Check sheet for the drawn part. Datum: minimum x, y, z corner. Units: mm. Coordinates: 2 decimals unless noted, no trailing zeros. Loops run counter-clockwise (first coordinate to the right, second up) from the corner with the lowest first, then second, coordinate; pieces in that order, holes last. Notation, with made-up numbers: (23.5, 4) - (30.5, 4) arc R18 cw to (30.5, 18) - close; hole circle Ø7 at (71, 65). An arc over 180 degrees is marked (long way). Answer as CSV lines item,"result". Start each with the question number.
1. Cross-section at B-B (y = 66). Enter the section's corners in (x, z).
2. Cross-section at C-C (z = 530). Enter the section's corners in (x, y), plus the area to 3 significant figures.
3. Cross-section at D-D (y = 212). Enter the section's corners in (x, z).
4. Gauge pin test, flat ends, axial feed: P1, Ø12.5, axis at x = 72.5, y = 177, coming from the +Z side; P2, Ø12, axis at x = 364.5, y = 23, coming from the -Z side; P3, Ø15, axis at x = 171.5, y = 196, coming from the +Z side. Record the tip position at first contact, or that the pin passes through.
5. Material ranges on line 1 (X direction, y = 44.5, z = 597.5); line 2 (X direction, y = 145.5, z = 645.5); line 3 (Z direction, x = 68.5, y = 183.5), recorded low to high. Write a range as [from, to].
6. Cross-section at A-A (x = 52). Enter the section's corners in (y, z), plus the area to 3 significant figures.
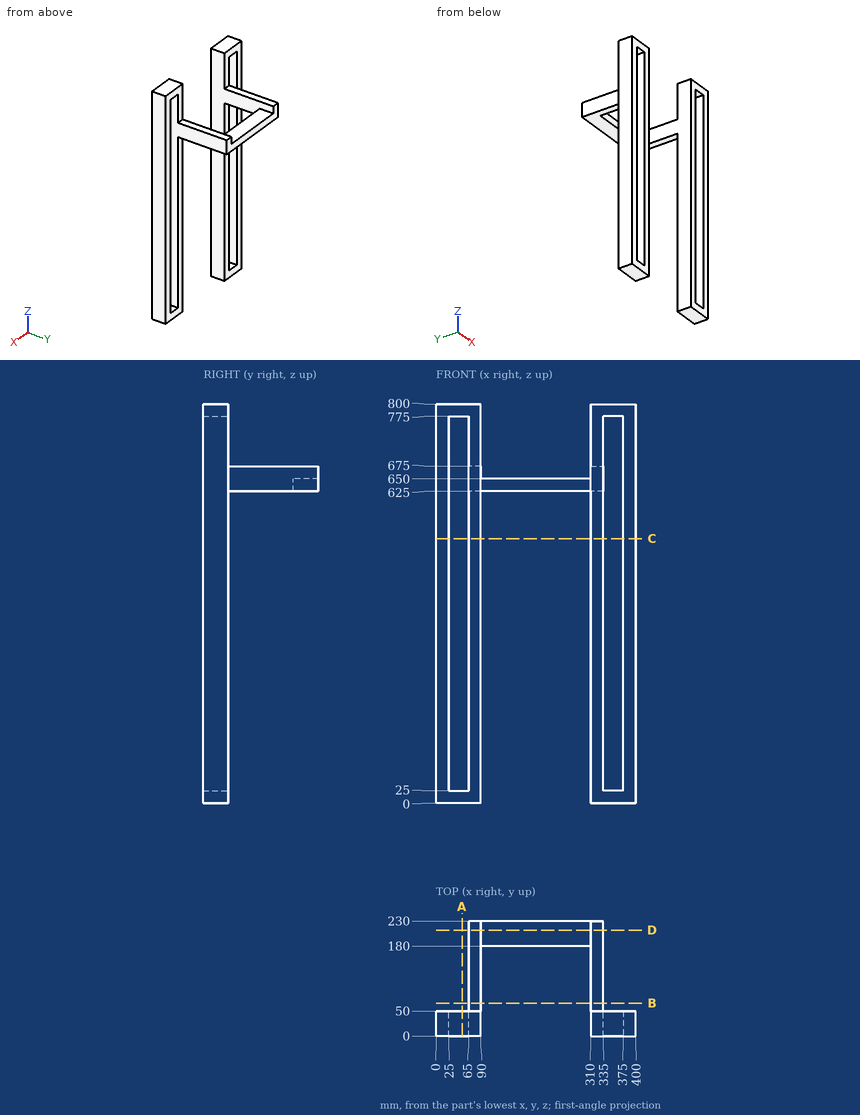
Values follow:
1,outline,"(65, 625) - (90, 625) - (90, 675) - (65, 675) - close; (310, 625) - (335, 625) - (335, 675) - (310, 675) - close"
2,outline,"(0, 0) - (25, 0) - (25, 50) - (0, 50) - close; (65, 0) - (90, 0) - (90, 50) - (65, 50) - close; (310, 0) - (335, 0) - (335, 50) - (310, 50) - close; (375, 0) - (400, 0) - (400, 50) - (375, 50) - close"
2,area,"5,000 mm²"
3,outline,"(65, 625) - (335, 625) - (335, 675) - (310, 675) - (310, 650) - (90, 650) - (90, 675) - (65, 675) - close"
4,P1,"stops at z = 675"
4,P2,"stops at z = 0"
4,P3,"stops at z = 650"
5,line 1,"x = [0, 25], [65, 90], [310, 335], [375, 400]"
5,line 2,"x = [65, 90], [310, 335]"
5,line 3,"z = [625, 675]"
6,outline,"(0, 0) - (50, 0) - (50, 25) - (0, 25) - close; (0, 775) - (50, 775) - (50, 800) - (0, 800) - close"
6,area,"2,500 mm²"
